For this review, use the dimensioned drawing (mm, ordinates from the lowest corner) and the shaded views. Round coordinates to 2 decimals unless told otherwise and drop trailing zeros. Write each loop counter-clockwise with the first axis right and the second up, starting at its lowest first coordinate (ties: lowest second). Pieces come first, ordered by that corner, then holes. Notation, with made-up numbers: (-5, -16.75) -> (40, -16.75) arc R14 ccw to (40, 8.25) -> close; hole circle Ø11 at (-38.5, 39). An arc over 180 degrees is marked (long way). Answer as CSV lines item,"result". Start each with the question number.
Item 1: Mouldability with a two-part tool opening along Y and no side actions: class the marked faces 1, 2, 3 and 4 as +Y half, -Y half, draft (parallel to the pull), parting line (faces both ways), or undercut.
Item 2: Wall thickness on probe 1 along X at (y, z) = (6, 6.5); probe 2 along Y at (x, z) = (10, 6.75); probe 3 along Y at (x, z) = (50.5, 12.25): over which ranges is each line inside the solid? List them lowest first. Write a range as from..to.
Item 3: Take a section at C-C on z = 11.25. Give the boundary of the cut face in (x, y).
Item 4: Take a section at B-B on x = 10. Give the boundary of the cut face in (y, z), then the cut area to 3 significant figures.
Item 5: Take a section at D-D on x = 23.5. Give the boundary of the cut face in (y, z), then the cut area to 3 significant figures.
Item 6: For pin 1 Ø1.5 at (y, z) = (41, 2) entering from -X; pin 2 Ø3 at (x, y) = (11, 36.5) entering from +Z, all flat-tipped, find the tip position at first contact; note any pin that passes through.
Item 7: Take a section at A-A on y = 45. Give the boundary of the cut face in (x, z), then the cut area to 3 significant figures.
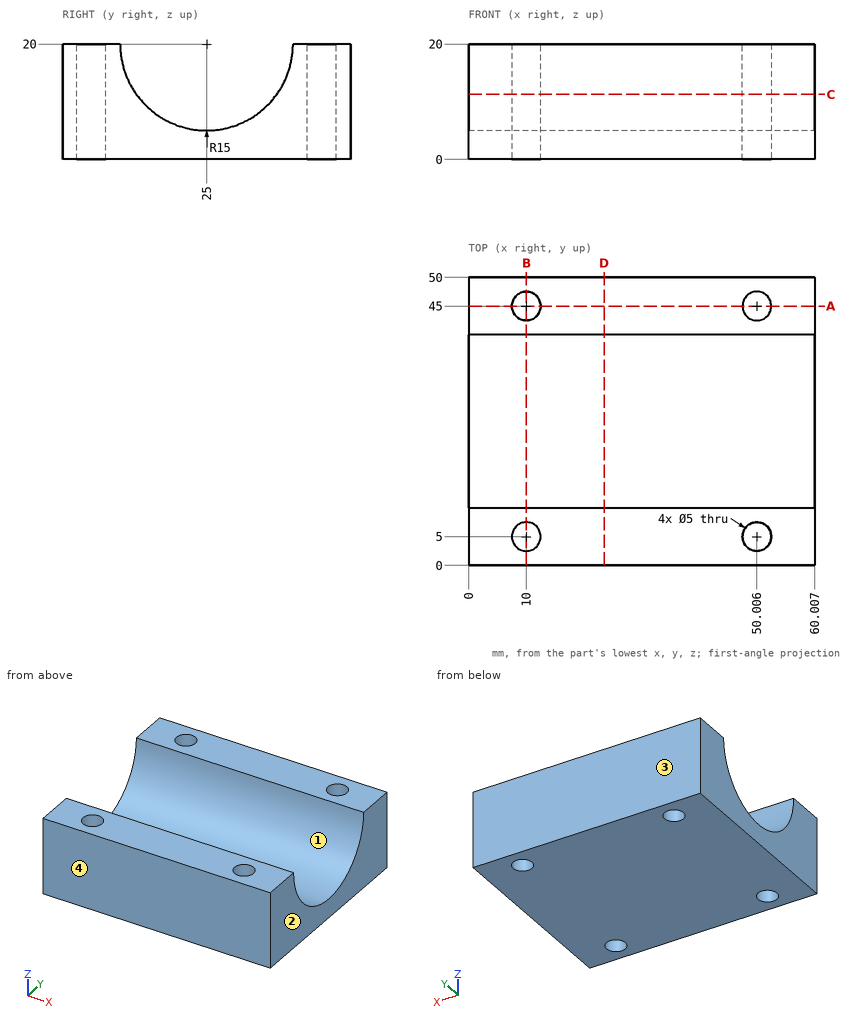
Output values:
1,face 1,"undercut"
1,face 2,"draft"
1,face 3,"+Y half"
1,face 4,"-Y half"
2,probe 1,"x = 0..7.71, 12.29..47.71, 52.3..60.01"
2,probe 2,"y = 0..2.5, 7.5..17.97, 32.03..42.5, 47.5..50"
2,probe 3,"y = 0..2.55, 7.45..12.16, 37.84..42.55, 47.45..50"
3,outline,"(0, 0) -> (60.01, 0) -> (60.01, 12.82) -> (0, 12.82) -> close; (0, 37.18) -> (60.01, 37.18) -> (60.01, 50) -> (0, 50) -> close; hole circle Ø5 at (10, 5); hole circle Ø5 at (10, 45); hole circle Ø5 at (50.01, 5); hole circle Ø5 at (50.01, 45)"
4,outline,"(0, 0) -> (2.5, 0) -> (2.5, 20) -> (0, 20) -> close; (7.5, 0) -> (42.5, 0) -> (42.5, 20) -> (40, 20) arc R15 cw to (10, 20) -> (7.5, 20) -> close; (47.5, 0) -> (50, 0) -> (50, 20) -> (47.5, 20) -> close"
4,area,"447 mm^2"
5,outline,"(0, 0) -> (50, 0) -> (50, 20) -> (40, 20) arc R15 cw to (10, 20) -> (0, 20) -> close"
5,area,"647 mm^2"
6,pin 1,"stops at x = 0"
6,pin 2,"stops at z = 12.52"
7,outline,"(0, 0) -> (7.5, 0) -> (7.5, 20) -> (0, 20) -> close; (12.5, 0) -> (47.51, 0) -> (47.51, 20) -> (12.5, 20) -> close; (52.51, 0) -> (60.01, 0) -> (60.01, 20) -> (52.51, 20) -> close"
7,area,"1,000 mm^2"
